Build history of the part. All positions in model axes, mm. A direction names the side the tool comes from. Give positions to 0.01 mm unless a question says otherwise; leave off trailing zeros. Order: outer loops, then holes, each group sorted by start corner. A loop starts at its lowest first (then second) coordinate and runs counter-clockwise, first axis right, second up. Notation, with made-up numbers: (28.5, 2.25) - (56.5, 2.25) arc R38 cw to (56.5, 41.25) - close; hole circle Ø2 at (16, -40). An arc over 180 degrees is marked (long way). One line per item, written item: value.
```python
from build123d import *

# Parameters (mm, degrees)
SM_BASE_FLANGE_1_DEPTH = 100
CUT_EXTRUDE_1_DEPTH    = 102.727577382
PATTERN_LINEAR_6_COUNT = 4
PATTERN_LINEAR_6_PITCH = 25


# Sheet-metal steps are written as plain solids
with BuildPart() as part:
    # Sketch 1 → Базовая кромка1 (new body)
    with BuildSketch(Plane(origin=(0, 0, 0), x_dir=(0, 0, -1), z_dir=(1, 0, 0))):
        with BuildLine():
            Line((-17.5, 6.5), (-14.5, 6.5))
            ThreePointArc((-14.5, 6.5), (-13.792893219, 6.207106781), (-13.5, 5.5))
            Line((-13.5, 5.5), (-13.5, 2))
            ThreePointArc((-13.5, 2), (-12.914213562, 0.585786438), (-11.5, 0))
            Line((-11.5, 0), (11.5, 0))
            ThreePointArc((11.5, 0), (12.914213562, 0.585786438), (13.5, 2))
            Line((13.5, 2), (13.5, 5.5))
            ThreePointArc((13.5, 5.5), (13.792893219, 6.207106781), (14.5, 6.5))
            Line((14.5, 6.5), (17.5, 6.5))
            Line((17.5, 6.5), (17.5, 7.5))
            Line((17.5, 7.5), (14.5, 7.5))
            ThreePointArc((14.5, 7.5), (13.085786438, 6.914213562), (12.5, 5.5))
            Line((12.5, 5.5), (12.5, 2))
            ThreePointArc((12.5, 2), (12.207106781, 1.292893219), (11.5, 1))
            Line((11.5, 1), (-11.5, 1))
            ThreePointArc((-11.5, 1), (-12.207106781, 1.292893219), (-12.5, 2))
            Line((-12.5, 2), (-12.5, 5.5))
            ThreePointArc((-12.5, 5.5), (-13.085786438, 6.914213562), (-14.5, 7.5))
            Line((-14.5, 7.5), (-17.5, 7.5))
            Line((-17.5, 7.5), (-17.5, 6.5))
        make_face()
    extrude(amount=SM_BASE_FLANGE_1_DEPTH)

    # Эскиз6 → Вырез-Вытянуть1 (cut, through all)
    with BuildSketch(Plane(origin=(0, 1, 0), x_dir=(1, 0, 0), z_dir=(0, 1, 0))):
        with BuildLine():
            Line((6.65, 3.15), (18.35, 3.15))
            ThreePointArc((18.35, 3.15), (21.5, 0), (18.35, -3.15))
            Line((18.35, -3.15), (6.65, -3.15))
            ThreePointArc((6.65, -3.15), (3.5, 0), (6.65, 3.15))
        make_face()
    cut_extrude_1 = extrude(amount=-CUT_EXTRUDE_1_DEPTH, mode=Mode.SUBTRACT)

    # Линейный массив6: Вырез-Вытянуть1 ×4
    with Locations(*[(i * PATTERN_LINEAR_6_PITCH, 0, 0) for i in range(1, PATTERN_LINEAR_6_COUNT)]):
        add(cut_extrude_1, mode=Mode.SUBTRACT)


solid = part.part
```
(1) 3-axis set-ups, long thin cutter, end or side, ignore diameter. For faces 1 (the face through (49, 1, 0)), 2 (the face through (78.5, 0.5, 0.1)), 3 (the face through (49, 6.5, 16)), 4 (the face through (49, 4, -13.5)): which of +Z, -Z, +X, -X, +Y, -Y reach the whole face in a straight line?
Completed:
face 1: +X, -X, +Y
face 2: +Y, -Y
face 3: +Z, +X, -X, -Y
face 4: -Z, +X, -X, -Y
(2) Slice it at A-A, the plane x = 34.5. Give the cut face in (y, z), and give its area (3 significant figures).
Completed:
outline: (0, -11.5) arc R2 ccw to (2, -13.5) - (5.5, -13.5) arc R1 cw to (6.5, -14.5) - (6.5, -17.5) - (7.5, -17.5) - (7.5, -14.5) arc R2 ccw to (5.5, -12.5) - (2, -12.5) arc R1 cw to (1, -11.5) - (1, -3.15) - (0, -3.15) - close; (0, 3.15) - (1, 3.15) - (1, 11.5) arc R1 cw to (2, 12.5) - (5.5, 12.5) arc R2 ccw to (7.5, 14.5) - (7.5, 17.5) - (6.5, 17.5) - (6.5, 14.5) arc R1 cw to (5.5, 13.5) - (2, 13.5) arc R2 ccw to (0, 11.5) - close
area: 39.1 mm²
(3) Slice it at B-B, the plane y = 4.25. Give the cut face in (x, z), and give its area (3 significant figures).
Completed:
outline: (0, -13.5) - (100, -13.5) - (100, -12.5) - (0, -12.5) - close; (0, 12.5) - (100, 12.5) - (100, 13.5) - (0, 13.5) - close
area: 200 mm²
(4) Slice it at D-D, the plane x = 76. Give the cut face in (y, z), and give its area (3 significant figures).
Completed:
outline: (0, -11.5) arc R2 ccw to (2, -13.5) - (5.5, -13.5) arc R1 cw to (6.5, -14.5) - (6.5, -17.5) - (7.5, -17.5) - (7.5, -14.5) arc R2 ccw to (5.5, -12.5) - (2, -12.5) arc R1 cw to (1, -11.5) - (1, 11.5) arc R1 cw to (2, 12.5) - (5.5, 12.5) arc R2 ccw to (7.5, 14.5) - (7.5, 17.5) - (6.5, 17.5) - (6.5, 14.5) arc R1 cw to (5.5, 13.5) - (2, 13.5) arc R2 ccw to (0, 11.5) - close
area: 45.4 mm²
(5) Pull direction Z, two halves, no side cores. Call faces 5 (the face through (49.3, 0.6, 12.93)), 6 (the face through (49.3, 0.57, -12.9)), 7 (the face through (49.3, 6.93, -13.1)), 8 (the face through (49, 0, 0)): +Z half, -Z half, draft (parallel to the pull), parting line (faces both ways), or undercut.
Completed:
face 5: +Z half
face 6: -Z half
face 7: undercut
face 8: draft
(6) Drill centre lines: line 1 (Z direction, x = 10, y = 5.25); line 2 (Y direction, x = 85.5, z = 16); line 3 (Y direction, x = 74, z = 1). Where is each one in solid material? Low to high.
Completed:
line 1: -13.5 to -12.5, 12.5 to 13.5
line 2: 6.5 to 7.5
line 3: 0 to 1
(7) Pin check, flat tips, straight feed: P1, Ø0.5, axis at x = 61.5, y = 0.5, coming from the -Z side; P2, Ø0.8, axis at x = 37.5, y = 0.5, coming from the +Z side; P3, Ø4, axis at x = 40.5, y = 4, coming from the -Z side; P4, Ø2, axis at y = 2.5, z = -1.5, coming from the +X side. Stop position of each tip, or through.
Completed:
P1: z = -13.06
P2: z = 13.17
P3: z = -13.63
P4: through
(8) Slice it at C-C, the plane z = 0. Give the cut face in (x, y).
Completed:
outline: (0, 0) - (3.5, 0) - (3.5, 1) - (0, 1) - close; (21.5, 0) - (28.5, 0) - (28.5, 1) - (21.5, 1) - close; (46.5, 0) - (53.5, 0) - (53.5, 1) - (46.5, 1) - close; (71.5, 0) - (78.5, 0) - (78.5, 1) - (71.5, 1) - close; (96.5, 0) - (100, 0) - (100, 1) - (96.5, 1) - close
